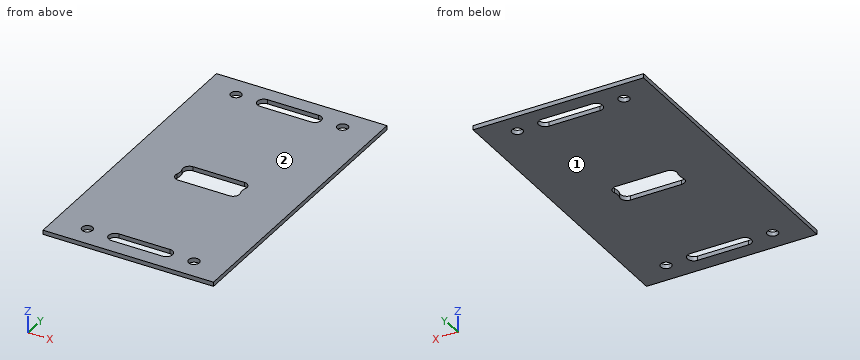
```python
from build123d import *

# Parameters (mm, degrees)
SKETCH1_W           = 40
SKETCH1_H           = 70
SKETCH1_R           = 1.25
BOSS_EXTRUDE1_DEPTH = 1
CUT_EXTRUDE1_DEPTH  = 41.323690307
FILLET1_R           = 3


with BuildPart() as part:
    # Sketch1 → Boss-Extrude1 (new body)
    with BuildSketch(Plane.XY):
        Rectangle(SKETCH1_W, SKETCH1_H)
        with Locations((-12.5, 30)):
            Circle(SKETCH1_R, mode=Mode.SUBTRACT)
        with Locations((12.5, 30)):
            Circle(SKETCH1_R, mode=Mode.SUBTRACT)
        with Locations((-12.5, -30)):
            Circle(SKETCH1_R, mode=Mode.SUBTRACT)
        with Locations((12.5, -30)):
            Circle(SKETCH1_R, mode=Mode.SUBTRACT)
    extrude(amount=BOSS_EXTRUDE1_DEPTH)

    # Sketch2 → Cut-Extrude1 (cut, through all)
    with BuildSketch(Plane.XY.offset(1)):
        with BuildLine():
            Line((-6, 31.5), (6, 31.5))
            ThreePointArc((6, 31.5), (7.5, 30), (6, 28.5))
            Line((6, 28.5), (-6, 28.5))
            ThreePointArc((-6, 28.5), (-7.5, 30), (-6, 31.5))
        make_face()
        with BuildLine():
            Line((-6, 1.5), (6, 1.5))
            ThreePointArc((6, 1.5), (7.5, 0), (6, -1.5))
            ThreePointArc((6, -1.5), (7.5, -3), (6, -4.5))
            Line((6, -4.5), (-6, -4.5))
            ThreePointArc((-6, -4.5), (-7.5, -3), (-6, -1.5))
            ThreePointArc((-6, -1.5), (-7.5, 0), (-6, 1.5))
        make_face()
        with BuildLine():
            Line((-6, -28.5), (6, -28.5))
            ThreePointArc((6, -28.5), (7.5, -30), (6, -31.5))
            Line((6, -31.5), (-6, -31.5))
            ThreePointArc((-6, -31.5), (-7.5, -30), (-6, -28.5))
        make_face()
    extrude(amount=-CUT_EXTRUDE1_DEPTH, mode=Mode.SUBTRACT)

    # Fillet1
    fillet1_edges = [part.edges().sort_by_distance(p)[0] for p in [
        (-6, -1.5, 0.5),
        (6, -1.5, 0.5),
    ]]
    fillet(fillet1_edges, radius=FILLET1_R)


solid = part.part
```
Build history of the part. All positions in model axes, mm. Face numbers are marked on the shaded views. Round coordinates to 2 decimals unless told otherwise and drop trailing zeros. Write each loop counter-clockwise with the first axis right and the second up, starting at its lowest first coordinate (ties: lowest second). Pieces come first, ordered by that corner, then holes.
1) Band-saw the part on B-B, the plane x = 0. List the corners of the cut face in (y, z), and give its area (3 significant figures).
2) Mould opens along Z. For the marked faces 1 and 2 say: +Z half, -Z half, draft (parallel to the pull), parting line (faces both ways), or undercut.
3) Band-saw the part on A-A, the plane x = -12.5. List the corners of the cut face in (y, z), and give its area (3 significant figures).
4) Drill centre lines: probe 1 along Y at (x, z) = (-12.5, 0.5); probe 2 along Y at (x, z) = (0.5, 0.5); probe 3 along Y at (x, z) = (13, 0.1). Where is each one in solid material? Low to high.
5) Band-saw the part on C-C, the plane z = 0.6. Give the number of separate pieces and of enclosed holes in the cut face, and give its area (3 significant figures).
Ans:
1. outline: (-35, 0) - (-31.5, 0) - (-31.5, 1) - (-35, 1) - close; (-28.5, 0) - (-4.5, 0) - (-4.5, 1) - (-28.5, 1) - close; (1.5, 0) - (28.5, 0) - (28.5, 1) - (1.5, 1) - close; (31.5, 0) - (35, 0) - (35, 1) - (31.5, 1) - close
1. area: 58.0 mm2
2. face 1: -Z half
2. face 2: +Z half
3. outline: (-35, 0) - (-31.25, 0) - (-31.25, 1) - (-35, 1) - close; (-28.75, 0) - (28.75, 0) - (28.75, 1) - (-28.75, 1) - close; (31.25, 0) - (35, 0) - (35, 1) - (31.25, 1) - close
3. area: 65.0 mm2
4. probe 1: y = -35 to -31.25, -28.75 to 28.75, 31.25 to 35
4. probe 2: y = -35 to -31.5, -28.5 to -4.5, 1.5 to 28.5, 31.5 to 35
4. probe 3: y = -35 to -31.15, -28.85 to 28.85, 31.15 to 35
5. separate pieces: 1
5. enclosed holes: 7
5. area: 2,610 mm2
